Design review of the part built by this model. Coordinates are the model's own, in mm. A direction names the side the tool comes from. Coordinates: 2 decimals unless noted, no trailing zeros. Loops run counter-clockwise (first coordinate to the right, second up) from the corner with the lowest first, then second, coordinate; pieces in that order, holes last. Notation, with made-up numbers: (48, 59) -> (52, 59) arc R21 cw to (52, 64) -> close; hole circle Ø5 at (35.5, -5.75). An arc over 180 degrees is marked (long way). Use a Markdown table: item, result. Add a question column.
Q1. For probe 1 along Y at (x, z) = (25.4, 2.3) (3 decimals); probe 2 along Y at (x, z) = (7, 32.5); probe 3 along X at (y, z) = (-25, 2), list the stretches that pass through material, from the lowest coordinate up.
Q2. Take a section at A-A on x = -25.4. Write out the cut boundary in (y, z) (3 decimals).
Q3. Take a section at B-B on z = 35. Write out the cut boundary in (x, y).
Q4. For faces 1 (the face through (26.381, 23.515, 1.565)), 2 (the face through (-1, 49, 26)), list the 3-axis set-ups (+Z, -Z, +X, -X, +Y, -Y) from which the entire face can be reached by the end or side of a thin tool; tool diameter is ignored.
Q5. Take a section at D-D on y = 0. Write out the cut boundary in (x, z) (3 decimals).
Q6. Draft analysis for pull direction Y (two halves, no side actions). For faces 3 (the face through (-49.3, 22.9, 50.038)), 4 (the face through (-1, 52, 26)), 5 (the face through (-12, 1, 0)), 6 (the face through (-49, -1, 26)), state which applies: pulls with the +Y half, pulls with the -Y half, needs draft (parallel to the pull), parting line crosses it, or undercut.
Q7. Clearance check with flat-ended pins moving along their axes: pin 1 Ø11.5 at (x, y) = (0, 0) entering from -Z; pin 2 Ø7 at (x, y) = (25.4, -25.4) entering from +Z (3 decimals). State where each tip first meets the part, or that it passes through.
from build123d import *

# Parameters (mm, degrees)
SKETCH_W      = 104
SKETCH_H      = 104
SKETCH_R      = 2.125
SKETCH_R_2    = 6.35
PAD_DEPTH     = 3.175
SKETCH003_W   = 104
SKETCH003_H   = 104
SKETCH003_W_2 = 98
SKETCH003_H_2 = 98
PAD002_DEPTH  = 46.863
SKETCH004_W   = 104
SKETCH004_H   = 104
SKETCH004_W_2 = 101.968
SKETCH004_H_2 = 101.968
PAD003_DEPTH  = 2


with BuildPart() as part:
    # Sketch → Pad (new body)
    with BuildSketch(Plane.XY):
        Rectangle(SKETCH_W, SKETCH_H)
        with Locations((-25.399999, 25.399999)):
            Circle(SKETCH_R, mode=Mode.SUBTRACT)
        with Locations((25.399999, 25.399999)):
            Circle(SKETCH_R, mode=Mode.SUBTRACT)
        with Locations((25.399999, -25.399999)):
            Circle(SKETCH_R, mode=Mode.SUBTRACT)
        with Locations((-25.399999, -25.399999)):
            Circle(SKETCH_R, mode=Mode.SUBTRACT)
        Circle(SKETCH_R_2, mode=Mode.SUBTRACT)
    extrude(amount=PAD_DEPTH)

    # Sketch003 (on Face11 of Pad) → Pad002 (join)
    with BuildSketch(Plane.XY.offset(3.175)):
        Rectangle(SKETCH003_W, SKETCH003_H)
        Rectangle(SKETCH003_W_2, SKETCH003_H_2, mode=Mode.SUBTRACT)
    extrude(amount=PAD002_DEPTH)

    # Sketch004 (on Face14 of Pad002) → Pad003 (join)
    with BuildSketch(Plane.XY.offset(50.038)):
        Rectangle(SKETCH004_W, SKETCH004_H)
        Rectangle(SKETCH004_W_2, SKETCH004_H_2, mode=Mode.SUBTRACT)
    extrude(amount=PAD003_DEPTH)


solid = part.part
Answer list:
| question | item | result |
|---|---|---|
| 1 | probe 1 | -52 to -27.525, -23.275 to 23.275, 27.525 to 52 |
| 1 | probe 2 | -52 to -49, 49 to 52 |
| 1 | probe 3 | -52 to -27.49, -23.31 to 23.31, 27.49 to 52 |
| 2 | outline | (-52, 0) -> (-27.525, 0) -> (-27.525, 3.175) -> (-49, 3.175) -> (-49, 50.038) -> (-50.984, 50.038) -> (-50.984, 52.038) -> (-52, 52.038) -> close; (-23.275, 0) -> (23.275, 0) -> (23.275, 3.175) -> (-23.275, 3.175) -> close; (27.525, 0) -> (52, 0) -> (52, 52.038) -> (50.984, 52.038) -> (50.984, 50.038) -> (49, 50.038) -> (49, 3.175) -> (27.525, 3.175) -> close |
| 3 | outline | (-52, -52) -> (52, -52) -> (52, 52) -> (-52, 52) -> close; hole (-49, -49) -> (49, -49) -> (49, 49) -> (-49, 49) -> close |
| 4 | face 1 | +Z, -Z |
| 4 | face 2 | +Z |
| 5 | outline | (-52, 0) -> (-6.35, 0) -> (-6.35, 3.175) -> (-49, 3.175) -> (-49, 50.038) -> (-50.984, 50.038) -> (-50.984, 52.038) -> (-52, 52.038) -> close; (6.35, 0) -> (52, 0) -> (52, 52.038) -> (50.984, 52.038) -> (50.984, 50.038) -> (49, 50.038) -> (49, 3.175) -> (6.35, 3.175) -> close |
| 6 | face 3 | undercut |
| 6 | face 4 | pulls with the +Y half |
| 6 | face 5 | needs draft |
| 6 | face 6 | undercut |
| 7 | pin 1 | through |
| 7 | pin 2 | z = 3.175 |
